Part model, mm, in its own coordinate system. Face numbers are marked on the shaded views. Give positions to 0.01 mm unless a question says otherwise; leave off trailing zeros. Write each loop counter-clockwise with the first axis right and the second up, starting at its lowest first coordinate (ties: lowest second). Pieces come first, ordered by that corner, then holes. Notation, with made-up numbers: M 65,69 L 72,69 A21 ccw 72,83 Z; hole C 17.25,22 d4. An arc over 180 degrees is marked long. Answer as CSV lines item,"result". Start each with the question number.
Item 1: Two-plate mould, pull along X, no slides. Class the marked faces 1 and 2: +X half, -X half, draft (parallel to the pull), parting line (faces both ways), or undercut.
Item 2: Band-saw the part on D-D, the plane y = 27.5. List the corners of the cut face in (x, z).
Item 3: Wall check: L1, parallel to X at y = 76.5, z = -1; L2, parallel to Y at x = -16.5, z = 10; L3, parallel to X at y = 10, z = -6.5. Give the ranges that are in metal, low to high. Write a range as from..to.
Item 4: Band-saw the part on B-B, the plane x = 0. List the corners of the cut face in (y, z), then the cut area to 3 significant figures.
Item 5: Band-saw the part on C-C, the plane x = -7. List the corners of the cut face in (y, z).
Item 6: Pin check, flat tips, straight feed: pin 1 (3 mm diameter, centred on x = 17, z = -11.5, fed in from +Y); pin 2 (5 mm diameter, centred on x = -18.5, y = 64.5, fed in from -Z); pin 3 (2 mm diameter, centred on x = -7.5, y = 60, fed in from +Z); pin 4 (12 mm diameter, centred on x = 20.5, z = -21, fed in from -Y). Stop position of each tip, or through.
Item 7: Band-saw the part on A-A, the plane z = 0. List the corners of the cut face in (x, y).
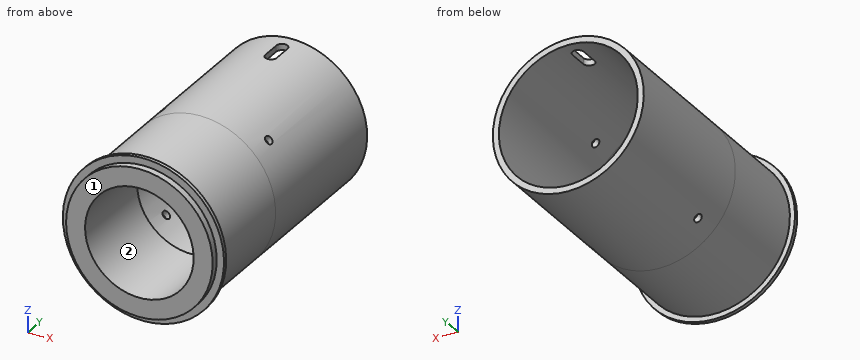
from build123d import *

# Parameters (mm, degrees)
SKETCH1_R                       = 24.5999
SKETCH1_R_2                     = 18.2245
BOSS_EXTRUDE1_DEPTH             = 4.3942
SKETCH2_R                       = 25.3365
SKETCH2_R_2                     = 18.2245
BOSS_EXTRUDE2_DEPTH             = 33.02
SKETCH15_R                      = 27.051
SKETCH15_R_2                    = 25.3365
BOSS_EXTRUDE3_DEPTH             = 1.27
SKETCH18_R                      = 25.3365
SKETCH18_R_2                    = 23.3045
BOSS_EXTRUDE5_DEPTH             = 53.34
CUT_EXTRUDE2_DEPTH              = 10.16
F_35_0_11_DIAMETER_HOLE1_REACH  = 112.817
F_35_0_11_DIAMETER_HOLE1_BORE_R = 1.397
CIRPATTERN1_COUNT               = 4
MOVE_FACE1_BY                   = 2.032
MOVE_FACE2_BY                   = 5.08


with BuildPart() as part:
    # Sketch1 → Boss-Extrude1 (new body)
    with BuildSketch(Plane(origin=(0, 0, 0), x_dir=(1, 0, 0), z_dir=(0, 1, 0))):
        with Locations(Location((0, 0, 0), (0, 0, 270))):
            Circle(SKETCH1_R)
        with Locations(Location((0, 0, 0), (0, 0, 270))):
            Circle(SKETCH1_R_2, mode=Mode.SUBTRACT)
    extrude(amount=BOSS_EXTRUDE1_DEPTH)

    # Sketch2 → Boss-Extrude2 (add)
    with BuildSketch(Plane(origin=(0, 4.3942, 0), x_dir=(1, 0, 0), z_dir=(0, 1, 0))):
        with Locations(Location((0, 0, 0), (0, 0, 270))):
            Circle(SKETCH2_R)
        with Locations(Location((0, 0, 0), (0, 0, 270))):
            Circle(SKETCH2_R_2, mode=Mode.SUBTRACT)
    extrude(amount=BOSS_EXTRUDE2_DEPTH)

    # Sketch15 → Boss-Extrude3 (add)
    with BuildSketch(Plane.XZ.offset(-4.3942)):
        with Locations(Location((0, 0, 0), (0, 0, 270))):
            Circle(SKETCH15_R)
        with Locations(Location((0, 0, 0), (0, 0, 270))):
            Circle(SKETCH15_R_2, mode=Mode.SUBTRACT)
    extrude(amount=-BOSS_EXTRUDE3_DEPTH)

    # Sketch18 → Boss-Extrude5 (add)
    with BuildSketch(Plane(origin=(0, 37.4142, 0), x_dir=(1, 0, 0), z_dir=(0, 1, 0))):
        with Locations(Location((0, 0, 0), (0, 0, 90))):
            Circle(SKETCH18_R)
        with Locations(Location((0, 0, 0), (0, 0, 270))):
            Circle(SKETCH18_R_2, mode=Mode.SUBTRACT)
    extrude(amount=BOSS_EXTRUDE5_DEPTH)

    # Sketch19 → Cut-Extrude2 (cut)
    with BuildSketch(Plane.XY.offset(25.3365)):
        with BuildLine():
            Line((1.905, 85.025248354), (1.905, 78.649848354))
            ThreePointArc((1.905, 78.649848354), (0, 76.744848354), (-1.905, 78.649848354))
            Line((-1.905, 78.649848354), (-1.905, 85.025248354))
            ThreePointArc((-1.905, 85.025248354), (0, 86.930248354), (1.905, 85.025248354))
        make_face()
    extrude(amount=-CUT_EXTRUDE2_DEPTH, mode=Mode.SUBTRACT)

    # #35 (0.11) Diameter Hole1 bore → #35 (0.11) Diameter Hole1 (cut, up to next)
    with BuildSketch(Plane(origin=(-17.915610962, 0, 17.915610962), x_dir=(0, -1, 0), z_dir=(-0.7071067811865488, 0, 0.7071067811865464)), mode=Mode.PRIVATE) as f_35_0_11_diameter_hole1_sk1:
        with Locations((-46.3042, 0)):
            Circle(F_35_0_11_DIAMETER_HOLE1_BORE_R)
    f_35_0_11_diameter_hole1_tool1 = extrude(f_35_0_11_diameter_hole1_sk1.sketch, amount=-F_35_0_11_DIAMETER_HOLE1_REACH, mode=Mode.PRIVATE) & part.part
    f_35_0_11_diameter_hole1 = f_35_0_11_diameter_hole1_tool1.solids().sort_by_distance((-17.915611, 46.3042, 17.915611))[0]
    add(f_35_0_11_diameter_hole1, mode=Mode.SUBTRACT)

    # CirPattern1: #35 (0.11) Diameter Hole1 ×4 about axis
    cirpattern1_axis = Axis((0, 37.4142, 0), (0, -1, 0))
    for i in range(1, CIRPATTERN1_COUNT):
        add(f_35_0_11_diameter_hole1.rotate(cirpattern1_axis, i * 360 / CIRPATTERN1_COUNT), mode=Mode.SUBTRACT)

    # Move Face1: a face moved inward by 2.032
    extrude(part.faces().sort_by_distance((0, 0, 19.67992))[0], amount=MOVE_FACE1_BY, dir=(0, 1, 0), mode=Mode.SUBTRACT)

    # Move Face2: a face moved inward by 5.08
    extrude(part.faces().sort_by_distance((0, 37.4142, 18.6436))[0], amount=MOVE_FACE2_BY, dir=(0, -1, 0), mode=Mode.SUBTRACT)


solid = part.part
Output:
1,face 1,"draft"
1,face 2,"undercut"
2,outline,"C 0,0 d50.67; hole C 0,0 d36.45"
3,L1,"-25.32..-23.28, 23.28..25.32"
3,L2,"2.03..32.33"
3,L3,"-24.49..-17.03, 17.03..24.49"
4,outline,"M 2.03,-24.6 L 4.39,-24.6 L 4.39,-27.05 L 5.66,-27.05 L 5.66,-25.34 L 90.75,-25.34 L 90.75,-23.3 L 32.33,-23.3 L 32.33,-18.22 L 2.03,-18.22 Z; M 2.03,18.22 L 32.33,18.22 L 32.33,23.3 L 76.74,23.3 L 76.74,25.34 L 5.66,25.34 L 5.66,27.05 L 4.39,27.05 L 4.39,24.6 L 2.03,24.6 Z; M 86.93,23.3 L 90.75,23.3 L 90.75,25.34 L 86.93,25.34 Z"
4,area,"649 mm²"
5,outline,"M 2.03,-23.58 L 4.39,-23.58 L 4.39,-26.13 L 5.66,-26.13 L 5.66,-24.35 L 90.75,-24.35 L 90.75,-22.23 L 32.33,-22.23 L 32.33,-16.83 L 2.03,-16.83 Z; M 2.03,16.83 L 32.33,16.83 L 32.33,22.23 L 90.75,22.23 L 90.75,24.35 L 5.66,24.35 L 5.66,26.13 L 4.39,26.13 L 4.39,23.58 L 2.03,23.58 Z"
6,pin 1,"y = 32.33"
6,pin 2,"z = -19.65"
6,pin 3,"z = 24.49"
6,pin 4,"y = 2.03"
7,outline,"M -27.05,4.39 L -24.6,4.39 L -24.6,2.03 L -18.22,2.03 L -18.22,32.33 L -23.3,32.33 L -23.3,90.75 L -25.34,90.75 L -25.34,5.66 L -27.05,5.66 Z; M 18.22,2.03 L 24.6,2.03 L 24.6,4.39 L 27.05,4.39 L 27.05,5.66 L 25.34,5.66 L 25.34,90.75 L 23.3,90.75 L 23.3,32.33 L 18.22,32.33 Z"
